Check sheet for the drawn part. Datum: minimum x, y, z corner. Units: mm. Give positions to 0.01 mm unless a question says otherwise; leave off trailing zeros. Order: outer loops, then holes, each group sorted by start corner. A loop starts at its lowest first (then second) coordinate and runs counter-clockwise, first axis right, second up.
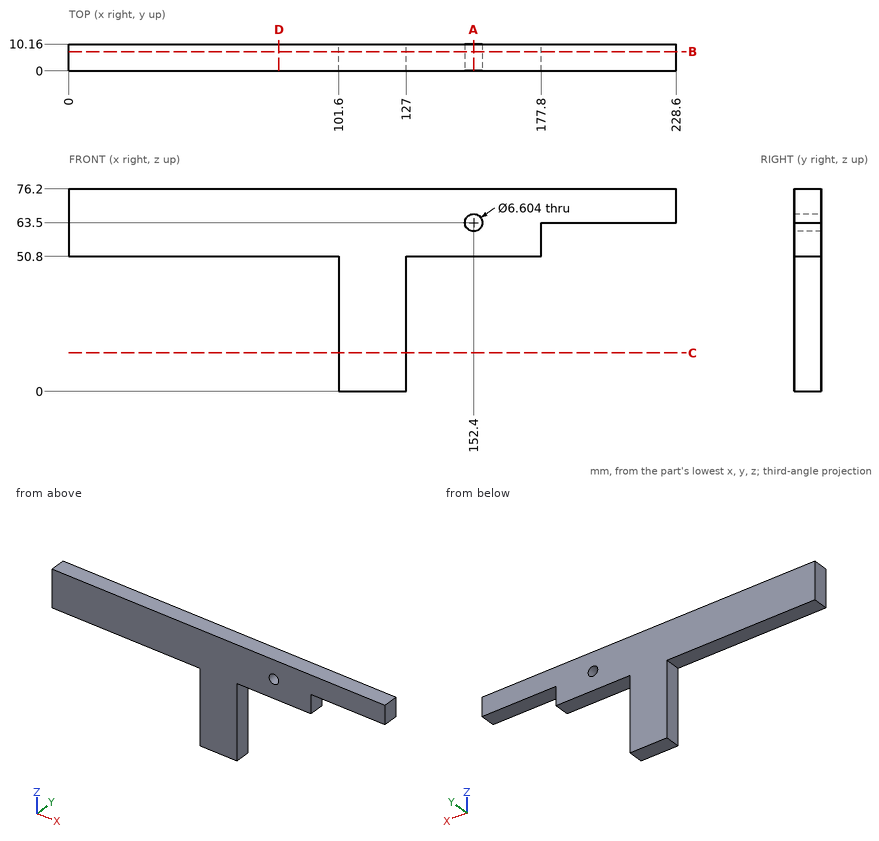
Item 1: Sectioned sample at D-D (x = 79). Enter the section's corners in (y, z).
Reported:
outline: (0, 50.8) - (10.16, 50.8) - (10.16, 76.2) - (0, 76.2) - close
Item 2: Gauge pin test, flat ends, axial feed: pin 1 (5 mm diameter, centred on y = 7.5, z = 36.5, fed in from +X); pin 2 (3 mm diameter, centred on y = 4, z = 56, fed in from +X); pin 3 (1 mm diameter, centred on y = 1.5, z = 26, fed in from -X). Record the tip position at first contact, or that the pin passes through.
Reported:
pin 1: stops at x = 127
pin 2: stops at x = 177.8
pin 3: stops at x = 101.6
Item 3: Sectioned sample at A-A (x = 152.4). Enter the section's corners in (y, z).
Reported:
outline: (0, 50.8) - (10.16, 50.8) - (10.16, 60.2) - (0, 60.2) - close; (0, 66.8) - (10.16, 66.8) - (10.16, 76.2) - (0, 76.2) - close
Item 4: Sectioned sample at B-B (y = 7.25). Enter the section's corners in (x, z), and give its area (3 significant figures).
Reported:
outline: (0, 50.8) - (101.6, 50.8) - (101.6, 0) - (127, 0) - (127, 50.8) - (177.8, 50.8) - (177.8, 63.5) - (228.6, 63.5) - (228.6, 76.2) - (0, 76.2) - close; hole circle Ø6.6 at (152.4, 63.5)
area: 6,420 mm2
Item 5: Scan lines: L1, parallel to Z at x = 152.4, y = 5.25; L2, parallel to Z at x = 80, y = 3.25; L3, parallel to X at y = 7.5, z = 53.5. Record each from-to range of solid material in increasing order.
Reported:
L1: z = 50.8 to 60.2, 66.8 to 76.2
L2: z = 50.8 to 76.2
L3: x = 0 to 177.8
Item 6: Sectioned sample at C-C (z = 14.5). Enter the section's corners in (x, y).
Reported:
outline: (101.6, 0) - (127, 0) - (127, 10.16) - (101.6, 10.16) - close
